Geometry check sheet. Reference: the model listing, model coordinates, mm. Face numbers are marked on the shaded views. Round coordinates to 2 decimals unless told otherwise and drop trailing zeros. Write each loop counter-clockwise with the first axis right and the second up, starting at its lowest first coordinate (ties: lowest second). Pieces come first, ordered by that corner, then holes. Notation, with made-up numbers: (66, 38) - (94, 38) arc R14 cw to (94, 45) - close; hole circle Ø10 at (8.25, -13.5). An arc over 180 degrees is marked (long way). Return JSON: item names as keys, results as strings.
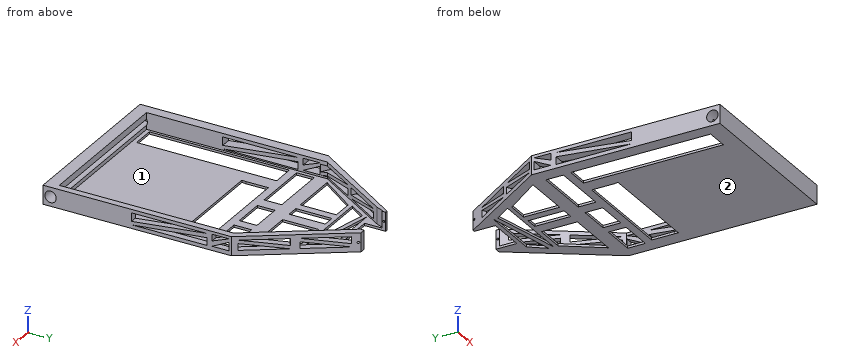
```python
from build123d import *

# Parameters (mm, degrees)
BOSS_EXTRUDE2_DEPTH      = 6.35
CUT_EXTRUDE1_DEPTH       = 5.588
CUT_EXTRUDE3_DEPTH       = 58.15
CUT_EXTRUDE4_DEPTH       = 58.15
CUT_EXTRUDE5_DEPTH       = 5.588
CUT_EXTRUDE6_DEPTH       = 5.588
SKETCH9_W                = 5.834897671
SKETCH9_H                = 6.35
CUT_EXTRUDE7_DEPTH       = 5.588
SKETCH14_W               = 35.347523306
SKETCH14_H               = 7.62
SKETCH14_W_2             = 7.5222908
SKETCH14_H_2             = 47.221578267
CUT_EXTRUDE15_DEPTH      = 1.762
CUT_EXTRUDE16_DEPTH      = 1.762
SKETCH16_W               = 19.137714492
SKETCH16_H               = 5.958224415
SKETCH16_W_2             = 10.658290022
SKETCH16_W_3             = 11.400659267
SKETCH16_W_4             = 3.957226521
SKETCH16_H_2             = 12.183905404
CUT_EXTRUDE18_DEPTH      = 1.762
SKETCH24_W               = 3.80459217
SKETCH24_H               = 5.588
CUT_EXTRUDE24_DEPTH      = 7.35
CUT_EXTRUDE25_DEPTH      = 11.684
SKETCH26_W               = 3.014165169
SKETCH26_H               = 5.588
CUT_EXTRUDE26_DEPTH      = 11.684
SKETCH28_R               = 0.333403054
CUT_EXTRUDE27_DEPTH      = 35.377669607
CUT_EXTRUDE27_DEPTH_BACK = 23.772330393
SKETCH29_R               = 1.924206534
CUT_EXTRUDE28_DEPTH      = 58.15


with BuildPart() as part:
    # Sketch1 → Boss-Extrude2 (new body)
    with BuildSketch(Plane.XY):
        Polygon((0, 0), (57.15, 0), (57.15, 63.5), (36.195, 95.25), (28.575, 95.25), (20.955, 95.25), (0, 63.5), align=None)
    extrude(amount=BOSS_EXTRUDE2_DEPTH)

    # Sketch2 → Cut-Extrude1 (cut)
    with BuildSketch(Plane.XY.offset(6.35)):
        Polygon((20.364000747, 91.616461208), (21.329039406, 94.01667417), (34.339089661, 94.01667417), (54.882736024, 62.961525589), (54.882736024, 4.173376451), (3.496365447, 4.173376451), (3.496365447, 65.109859062), align=None)
    extrude(amount=-CUT_EXTRUDE1_DEPTH, mode=Mode.SUBTRACT)

    # Sketch5 → Cut-Extrude3 (cut, through all)
    with BuildSketch(Plane(origin=(57.15, 0, 0), x_dir=(0, 0, -1), z_dir=(1, 0, 0))):
        Polygon((-5.197962118, 29.849901792), (-2.356915502, 29.849901792), (-5.197962118, 55.260698225), align=None)
        Polygon((-1.216346756, 29.849901792), (-1.216346756, 55.260698225), (-3.77743881, 55.260698225), align=None)
    extrude(amount=-CUT_EXTRUDE3_DEPTH, mode=Mode.SUBTRACT)

    # Sketch6 → Cut-Extrude4 (cut, through all)
    with BuildSketch(Plane(origin=(57.15, 0, 0), x_dir=(0, 0, -1), z_dir=(1, 0, 0))):
        Polygon((-5.412954005, 57.003118273), (-3.170845056, 57.003118273), (-5.412954005, 62.734975907), align=None)
        Polygon((-4.291899531, 62.734975907), (-1.412268241, 62.734975907), (-1.412268241, 57.003118273), align=None)
    extrude(amount=-CUT_EXTRUDE4_DEPTH, mode=Mode.SUBTRACT)

    # Sketch7 → Cut-Extrude5 (cut)
    with BuildSketch(Plane(origin=(69.002507662, 45.541655057, 0), x_dir=(0, 0, -1), z_dir=(0.834609407, 0.550842208, 0))):
        Polygon((-5.125103363, 23.517131124), (-5.125103363, 38.818816904), (-2.804754482, 38.818816904), align=None)
        Polygon((-3.964928922, 23.517131124), (-1.710138277, 23.517131124), (-1.710138277, 38.818816904), align=None)
        Polygon((-5.125103363, 41.600750711), (-5.125103363, 56.813922895), (-2.804754482, 56.813922895), align=None)
        Polygon((-3.964928922, 41.600750711), (-1.710138277, 41.600750711), (-1.710138277, 56.813922895), align=None)
    extrude(amount=-CUT_EXTRUDE5_DEPTH, mode=Mode.SUBTRACT)

    # Sketch8 → Cut-Extrude6 (cut)
    with BuildSketch(Plane(origin=(-29.193368626, 19.267623293, 0), x_dir=(0, 0, 1), z_dir=(-0.834609407, 0.550842208, 0))):
        Polygon((5.014666305, 54.401267981), (2.473695685, 54.401267981), (5.014666305, 69.338714317), align=None)
        Polygon((1.401941454, 54.401267981), (1.401941454, 69.338714317), (3.744180995, 69.338714317), align=None)
        Polygon((5.014666305, 71.297820033), (2.573061224, 71.297820033), (4.755204833, 85.214267299), align=None)
        Polygon((1.401941454, 71.297820033), (1.401941454, 85.214267299), (3.793863765, 85.214267299), align=None)
    extrude(amount=-CUT_EXTRUDE6_DEPTH, mode=Mode.SUBTRACT)

    # Sketch9 → Cut-Extrude7 (cut)
    with BuildSketch(Plane(origin=(0, 95.25, 0), x_dir=(1, 0, 0), z_dir=(0, 1, 0))):
        with Locations((28.446055603, -3.175)):
            Rectangle(SKETCH9_W, SKETCH9_H)
    extrude(amount=-CUT_EXTRUDE7_DEPTH, mode=Mode.SUBTRACT)

    # Sketch14 → Cut-Extrude15 (cut, through all)
    with BuildSketch(Plane.XY.offset(0.762)):
        with Locations((34.456497677, 49.047397654)):
            Rectangle(SKETCH14_W, SKETCH14_H)
        with Locations((8.166161846, 29.246608521)):
            Rectangle(SKETCH14_W_2, SKETCH14_H_2)
    extrude(amount=-CUT_EXTRUDE15_DEPTH, mode=Mode.SUBTRACT)

    # Sketch15 → Cut-Extrude16 (cut, through all)
    with BuildSketch(Plane.XY.offset(0.762)):
        Polygon((16.621939644, 43.865236106), (52.148781332, 43.865236106), (52.13025933, 45.237397654), (16.782736024, 45.237397654), align=None)
    extrude(amount=-CUT_EXTRUDE16_DEPTH, mode=Mode.SUBTRACT)

    # Sketch16 → Cut-Extrude18 (cut, through all)
    with BuildSketch(Plane.XY.offset(0.762)):
        with Locations((14.332787326, 58.472819058)):
            Rectangle(SKETCH16_W, SKETCH16_H)
        with Locations((33.188016104, 58.472819058)):
            Rectangle(SKETCH16_W_2, SKETCH16_H)
        with Locations((47.320715601, 58.472819058)):
            Rectangle(SKETCH16_W_3, SKETCH16_H)
        Polygon((49.98907512, 66.19967542), (41.620385968, 78.383580824), (31.6768604, 78.383580824), (31.6768604, 66.19967542), align=None)
        with Locations((25.880257832, 72.291628122)):
            Rectangle(SKETCH16_W_4, SKETCH16_H_2)
        Polygon((5.507881152, 66.19967542), (14.332787326, 78.383580824), (21.316943171, 78.383580824), (21.316943171, 66.19967542), align=None)
        Polygon((18.022227631, 85.25088415), (14.332787326, 79.783581396), (41.620385968, 79.783581396), align=None)
        Polygon((18.022227631, 86.733909891), (37.577072812, 86.733909891), (41.620385968, 81.514612422), align=None)
    extrude(amount=-CUT_EXTRUDE18_DEPTH, mode=Mode.SUBTRACT)

    # Sketch24 → Cut-Extrude24 (cut, through all)
    with BuildSketch(Plane(origin=(0, 0, 0), x_dir=(-1, 0, 0), z_dir=(0, 0, -1))):
        with Locations((-23.626310682, 92.456)):
            Rectangle(SKETCH24_W, SKETCH24_H)
    extrude(amount=-CUT_EXTRUDE24_DEPTH, mode=Mode.SUBTRACT)

    # Sketch25 → Cut-Extrude25 (cut)
    with BuildSketch(Plane(origin=(0, 0, 0), x_dir=(-1, 0, 0), z_dir=(0, 0, -1))):
        Polygon((-21.724014597, 89.662), (-21.724014597, 88.165353891), (-34.377669607, 88.165353891), (-34.377669607, 89.662), (-31.363504438, 89.662), align=None)
    extrude(amount=-CUT_EXTRUDE25_DEPTH, mode=Mode.SUBTRACT)

    # Sketch26 → Cut-Extrude26 (cut)
    with BuildSketch(Plane(origin=(0, 0, 0), x_dir=(-1, 0, 0), z_dir=(0, 0, -1))):
        with Locations((-32.870587023, 92.456)):
            Rectangle(SKETCH26_W, SKETCH26_H)
    extrude(amount=-CUT_EXTRUDE26_DEPTH, mode=Mode.SUBTRACT)

    # Sketch28 → Cut-Extrude27 (cut, two sides)
    with BuildSketch(Plane.ZY.offset(-34.377669607)) as cut_extrude27_sk:
        with Locations(Location((3.175, 94.604177073, 0), (0, 0, 90))):  # turned: the seam where the file's is
            Circle(SKETCH28_R)
    extrude(amount=CUT_EXTRUDE27_DEPTH, mode=Mode.SUBTRACT)
    extrude(cut_extrude27_sk.sketch, amount=-CUT_EXTRUDE27_DEPTH_BACK, mode=Mode.SUBTRACT)

    # Sketch29 → Cut-Extrude28 (cut, through all)
    with BuildSketch(Plane(origin=(57.15, 0, 0), x_dir=(0, 0, -1), z_dir=(1, 0, 0))):
        with Locations((-3.151671904, 2.54588231)):
            Circle(SKETCH29_R)
    extrude(amount=-CUT_EXTRUDE28_DEPTH, mode=Mode.SUBTRACT)


solid = part.part
```
(1) Gauge pin test, flat ends, axial feed: pin 1 (0.7 mm diameter, centred on x = 27, z = 5.5, fed in from +Y); pin 2 (3 mm diameter, centred on x = 12, y = 30, fed in from +Z); pin 3 (0.8 mm diameter, centred on x = 31, z = 0.5, fed in from +Y). Record the tip position at first contact, or that the pin passes through.
Response values:
{"pin 1": "stops at y = 4.17", "pin 2": "stops at z = 0.76", "pin 3": "stops at y = 88.17"}
(2) Section check A-A, the plane x = 30. Enter the section's corners in (y, z).
Response values:
{"outline": "(0, 0) - (43.87, 0) - (43.87, 0.76) - (4.17, 0.76) - (4.17, 2.13) arc R1.92 cw (long way) to (4.17, 4.18) - (4.17, 6.35) - (0, 6.35) - close; (52.86, 0) - (55.49, 0) - (55.49, 0.76) - (52.86, 0.76) - close; (61.45, 0) - (79.78, 0) - (79.78, 0.76) - (61.45, 0.76) - close; (82.48, 0) - (84.08, 0) - (84.08, 0.76) - (82.48, 0.76) - close; (86.73, 0) - (88.17, 0) - (88.17, 0.76) - (86.73, 0.76) - close"}
(3) Material ranges on line 1 along X through (y, z) = (28, 6); line 2 along X through (y, z) = (75.5, 0.5); line 3 along Y through (x, z) = (20, 0.5), recorded low to high. Write a range as [from, to].
Response values:
{"line 1": "x = [0, 3.5], [54.88, 57.15]", "line 2": "x = [7.92, 12.24], [21.32, 23.9], [27.86, 31.68], [43.6, 49.23]", "line 3": "y = [0, 43.87], [52.86, 55.49], [61.45, 66.2], [78.38, 79.78], [84.79, 86.3], [86.73, 93.8]"}
(4) Release check for a two-part mould opening along Y. For the marked faces 1 and 2 record: pulls with the +Y half, pulls with the -Y half, needs draft (parallel to the pull), parting line crosses it, or undercut.
Response values:
{"face 1": "undercut", "face 2": "needs draft"}
(5) Section check B-B, the plane x = 7.5. Give the number of separate pieces and of enclosed holes in the cut face, plus the area to 3 significant figures.
Response values:
{"separate pieces": "6", "enclosed holes": "0", "area": "37.6 mm^2"}
